Verification items for the finished model (mm, model axes). A direction names the side the tool comes from. Give positions to 0.01 mm unless a question says otherwise; leave off trailing zeros. Loops run counter-clockwise (first coordinate to the right, second up) from the corner with the lowest first, then second, coordinate; pieces in that order, holes last. Notation, with made-up numbers: M 37.5,22.25 L 47.5,22.25 A23 ccw 47.5,30.25 Z; hole C 79,12 d7. An arc over 180 degrees is marked long. Use CSV: the item, a comma, the result in double quotes.
from build123d import *

# Parameters (mm, degrees)
SKETCH_1_W      = 20
SKETCH_1_H      = 15
EXTRUDE_1_DEPTH = 5
EXTRUDE_2_DEPTH = 5


with BuildPart() as part:
    # 草图1 → 凸台-拉伸1 (new body)
    with BuildSketch(Plane.XY):
        with Locations((-4.771573604, 7.043147208)):
            Rectangle(SKETCH_1_W, SKETCH_1_H)
    extrude(amount=EXTRUDE_1_DEPTH)

    # 草图4 → 凸台-拉伸2 (add)
    with BuildSketch(Plane.XY.offset(5)):
        Polygon((-14.771573604, -0.456852792), (5.228426396, -0.456852792), (5.228426396, 4.543147208), (-9.771573604, 4.543147208), (-9.771573604, 9.543147208), (5.228426396, 9.543147208), (5.228426396, 14.543147208), (-14.771573604, 14.543147208), align=None)
    extrude(amount=EXTRUDE_2_DEPTH)


solid = part.part
(1) Mould release check, pull along Y, two halves, no side actions. Record for faces 3 (the flat face through (-9.772, 7, 7)), 4 (the flat face through (-5, -0.457, 5)), 5 (the flat face through (-14.772, 7, 5)): released by +Y, released by -Y, zero draft, split by the parting line, or undercut.
Calculated:
face 3,"undercut"
face 4,"released by -Y"
face 5,"zero draft"
(2) Scan lines: L1, parallel to Y at x = 3.75, z = 8.75; L2, parallel to X at y = 7.5, z = 8; L3, parallel to Z at x = -8.5, y = 7. Record each from-to range of solid material in increasing order. Write a range as from..to.
Calculated:
L1,"y = -0.46..4.54, 9.54..14.54"
L2,"x = -14.77..-9.77"
L3,"z = 0..5"
(3) Section check B-B on z = 9. Record the cut outline in (x, y), plus the area to 3 significant figures.
Calculated:
outline,"M -14.77,-0.46 L 5.23,-0.46 L 5.23,4.54 L -9.77,4.54 L -9.77,9.54 L 5.23,9.54 L 5.23,14.54 L -14.77,14.54 Z"
area,"225 mm²"
(4) Tool access check on faces 1 (the flat face through (-2, 9.543, 7)), 2 (the flat face through (5.228, 7, 4)). Record the directions out of +Z, -Z, +X, -X, +Y, -Y that give a thin tool (end or side, any length) a straight path to the whole face; none if there is none.
Calculated:
face 1,"+Z, +X"
face 2,"+Z, -Z, +X, +Y, -Y"
(5) Section check C-C on y = 5. Record the cut outline in (x, z).
Calculated:
outline,"M -14.77,0 L 5.23,0 L 5.23,5 L -9.77,5 L -9.77,10 L -14.77,10 Z"
(6) Section check A-A on x = -3. Record the cut outline in (y, z), plus the area to 3 significant figures.
Calculated:
outline,"M -0.46,0 L 14.54,0 L 14.54,10 L 9.54,10 L 9.54,5 L 4.54,5 L 4.54,10 L -0.46,10 Z"
area,"125 mm²"
